Model file for the job. Use its own axes, mm. Face numbers are marked on the shaded views. Give positions to 0.01 mm unless a question says otherwise; leave off trailing zeros. Write each loop counter-clockwise with the first axis right and the second up, starting at its lowest first coordinate (ties: lowest second). Pieces come first, ordered by that corner, then holes. Notation, with made-up numbers: (-35, 61.25) - (-21, 61.25) arc R9 ccw to (-21, 67.25) - close; hole circle Ø5 at (84, 30). An arc over 180 degrees is marked (long way). One line per item, written item: value. Start each with the question number.
(1) Mould opens along X. For the marked faces 1, 2 and 3 say: pulls with the +X half, pulls with the -X half, needs draft (parallel to the pull), parting line crosses it, or undercut.
(2) Cut at A-A, the plane y = -7. List the corners of the cut face in (x, z).
(3) Cut at B-B, the plane x = -33. List the corners of the cut face in (y, z).
(4) Cut at C-C, the plane z = 55. List the corners of the cut face in (x, y), and give its area (3 significant figures).
(5) Drop flat-ended pins along their axis: P1, Ø8, axis at x = 92.5, y = -12, coming from the -Z side; P2, Ø10, axis at x = 88, y = -2.5, coming from the -Z side; P3, Ø12, axis at y = -19.5, z = 48.5, coming from the -X side; P4, Ø13.5, axis at x = 95.73, z = 68.97, coming from the +Y side. Give the stop position or say it passes through.
(6) Probe L1, parallel to Z at x = 37.5, y = -22.25; L2, parallel to Z at x = 12, y = -21.25; L3, parallel to X at y = -2, z = -14. List the from-to ranges inside material, lowest first.
from build123d import *

# Parameters (mm, degrees)
F0_R     = 106.32546
F1_DEPTH = 25.4
F3_R     = 37.196049
F4_DEPTH = 25.401
F5_R     = 8.300114
F6_DEPTH = 25.4


with BuildPart() as f1:
    # F0 (on Front) → F1 (new body)
    with BuildSketch(Plane.XZ):
        with Locations((36.792137, 0)):
            Circle(F0_R)
    extrude(amount=F1_DEPTH)

    # F3 (on face) → F4 (cut, through all)
    with BuildSketch(Plane.XZ.offset(25.4)):
        with Locations((36.022916, -0.947487)):
            Circle(F3_R)
    extrude(amount=-F4_DEPTH, mode=Mode.SUBTRACT)

    # F5 (on face) → F6 (cut)
    with BuildSketch(Plane.XZ.offset(25.4)):
        with Locations((95.72994, 68.969317)):
            Circle(F5_R)
    extrude(amount=-F6_DEPTH, mode=Mode.SUBTRACT)


solid = f1.part
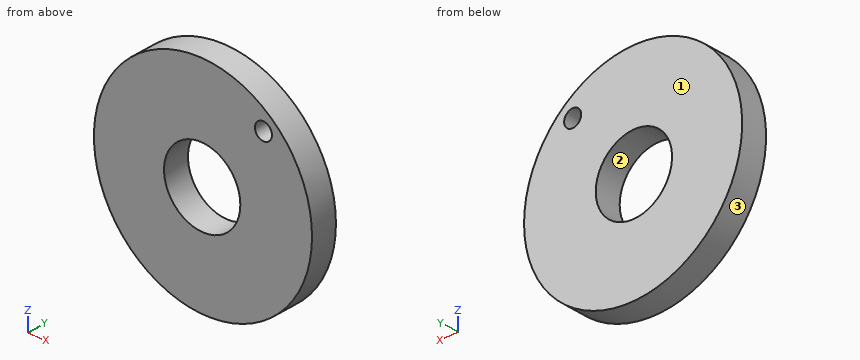
Answers follow:
1. face 1: needs draft
1. face 2: undercut
1. face 3: parting line crosses it
2. outline: circle Ø212.65 at (36.79, 0); hole circle Ø74.39 at (36.02, -0.95); hole circle Ø16.6 at (95.73, 68.97)
3. outline: (-25.4, -80.21) - (0, -80.21) - (0, 80.21) - (-25.4, 80.21) - close
4. outline: (-54.2, -25.4) - (127.79, -25.4) - (127.79, 0) - (-54.2, 0) - close
4. area: 4,620 mm²
5. P1: stops at z = -92.91
5. P2: stops at z = -95.76
5. P3: stops at x = -60.67
5. P4: passes through
6. L1: z = -106.32 to -38.11, 36.22 to 106.32
6. L2: z = -103.39 to -29.35, 27.45 to 103.39
6. L3: x = -68.61 to 1.19, 70.85 to 142.19
